```python
from build123d import *

# Parameters (mm, degrees)
SKETCH1_R                     = 16.891
BOSS_EXTRUDE1_DEPTH           = 3.175
F_2_CLEARANCE_HOLE1_D         = 2.4384
CIRPATTERN1_COUNT             = 6
F_3_CLEARANCE_HOLE1_OUTLINE_R = 1.397
F_3_CLEARANCE_HOLE1_DEPTH     = 3.175
SKETCH12_R                    = 9.144
CUT_EXTRUDE1_DEPTH            = 25.097559773


# Read off the part's stored shape, not the designer's step: #3 Clearance Hole1
with BuildPart() as part:
    # Sketch1 → Boss-Extrude1 (new body)
    with BuildSketch(Plane.XY):
        Circle(SKETCH1_R)
    extrude(amount=BOSS_EXTRUDE1_DEPTH)

    # #2 Clearance Hole1 (through all)
    with Locations(Plane.XY.offset(3.175)):
        with Locations((13.4874, 0)):
            f_2_clearance_hole1 = Hole(F_2_CLEARANCE_HOLE1_D / 2)

    # CirPattern1: #2 Clearance Hole1 ×6 about axis
    cirpattern1_axis = Axis((0, 0, 0), (0, 0, 1))
    for i in range(1, CIRPATTERN1_COUNT):
        add(f_2_clearance_hole1.rotate(cirpattern1_axis, i * 360 / CIRPATTERN1_COUNT), mode=Mode.SUBTRACT)

    # #3 Clearance Hole1 outline → #3 Clearance Hole1 (cut)
    with BuildSketch(Plane.XY):
        with Locations((-8, 8)):
            Circle(F_3_CLEARANCE_HOLE1_OUTLINE_R)
        with Locations((8, -8)):
            Circle(F_3_CLEARANCE_HOLE1_OUTLINE_R)
        with Locations((-8, -8)):
            Circle(F_3_CLEARANCE_HOLE1_OUTLINE_R)
        with Locations((8, 8)):
            Circle(F_3_CLEARANCE_HOLE1_OUTLINE_R)
    extrude(amount=F_3_CLEARANCE_HOLE1_DEPTH, mode=Mode.SUBTRACT)

    # Sketch12 → Cut-Extrude1 (cut, through all)
    with BuildSketch(Plane.XY.offset(3.175)):
        Circle(SKETCH12_R)
    extrude(amount=-CUT_EXTRUDE1_DEPTH, mode=Mode.SUBTRACT)


solid = part.part
```
Could you check a few things on this model? Use its own coordinates, in mm. Coordinates: 2 decimals unless noted, no trailing zeros. Order: outer loops, then holes, each group sorted by start corner. A loop starts at its lowest first (then second) coordinate and runs counter-clockwise, first axis right, second up. Notation, with made-up numbers: M -13.5,48 L 12.5,48 A30 cw 12.5,72 Z; hole C 69,35 d8. An arc over 180 degrees is marked long. Use a Markdown table: item, result. Add a question column.
Q1. I want a section at D-D on z = 1.25. Give the number of separate pieces and of enclosed holes in the cut face, then the cut area to 3 significant figures.
Q2. I want a section at A-A on y = 0. List the corners of the cut face in (x, z) for me (3 decimals), then the cut area to 3 significant figures.
Q3. I'm going to push flat-ended pins straight in: pin 1 (4.5 mm diameter, centred on x = -8, y = 8, fed in from +Z) (3 decimals); pin 2 (1 mm diameter, centred on x = -8, z = 1, fed in from +Y). Where does each tip first touch, or does it pass through?
Q4. If I drill on L1, parallel to Y at x = -7.5, z = 2.95; L2, parallel to Y at x = 0, z = 1.2; L3, parallel to Y at x = -8, z = 2.1, over which ranges is the centre line in solid material (lowest first)?
Q5. We'd pull the mould along X, two halves only. Please class faces 1 (the cylindrical face through (16.111, 5.074, 1.565)), 2 (the flat face through (0, -11, 0)), 3 (the cylindrical face through (7.87, -11.21, 1.57)): pulls with the +X half, pulls with the -X half, needs draft (parallel to the pull), parting line crosses it, or undercut.
Q6. I want a section at B-B on x = 0. List the corners of the cut face in (y, z) for me (3 decimals).
Q7. I want a section at C-C on y = 5. List the corners of the cut face in (x, z) for me (3 decimals), then the cut area to 3 significant figures.
Checked values:
| question | item | result |
|---|---|---|
| 1 | separate pieces | 1 |
| 1 | enclosed holes | 11 |
| 1 | area | 581 mm² |
| 2 | outline | M -16.891,0 L -14.707,0 L -14.707,3.175 L -16.891,3.175 Z; M -12.268,0 L -9.144,0 L -9.144,3.175 L -12.268,3.175 Z; M 9.144,0 L 12.268,0 L 12.268,3.175 L 9.144,3.175 Z; M 14.707,0 L 16.891,0 L 16.891,3.175 L 14.707,3.175 Z |
| 2 | area | 33.7 mm² |
| 3 | pin 1 | z = 3.175 |
| 3 | pin 2 | y = 15.13 |
| 4 | L1 | -15.13 to -12.64, -10.72 to -9.3, -6.7 to -5.23, 5.23 to 6.7, 9.3 to 10.72, 12.64 to 15.13 |
| 4 | L2 | -16.89 to -9.14, 9.14 to 16.89 |
| 4 | L3 | -14.88 to -9.4, -6.6 to -4.43, 4.43 to 6.6, 9.4 to 14.88 |
| 5 | face 1 | parting line crosses it |
| 5 | face 2 | needs draft |
| 5 | face 3 | undercut |
| 6 | outline | M -16.891,0 L -9.144,0 L -9.144,3.175 L -16.891,3.175 Z; M 9.144,0 L 16.891,0 L 16.891,3.175 L 9.144,3.175 Z |
| 7 | outline | M -16.134,0 L -7.656,0 L -7.656,3.175 L -16.134,3.175 Z; M 7.656,0 L 16.134,0 L 16.134,3.175 L 7.656,3.175 Z |
| 7 | area | 53.8 mm² |
